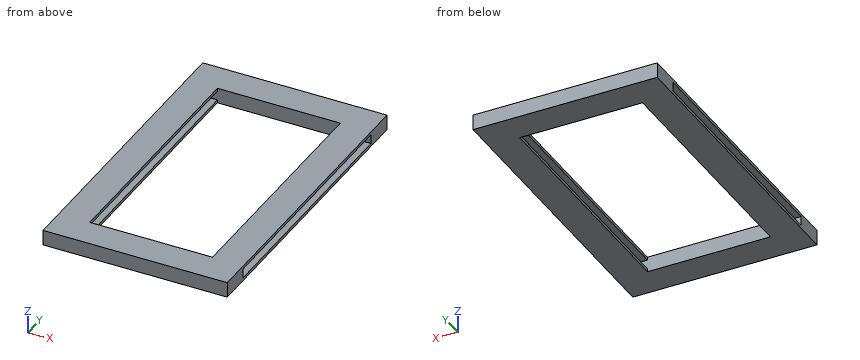
from build123d import *

# Parameters (mm, degrees)
CROQUIS1_W              = 60
CROQUIS1_H              = 100
SALIENTE_EXTRUIR1_DEPTH = 5
CROQUIS3_W              = 3
CROQUIS3_H              = 80
CORTAR_EXTRUIR2_DEPTH   = 60
CROQUIS4_W              = 40
CROQUIS4_H              = 80
CORTAR_EXTRUIR3_DEPTH   = 28


with BuildPart() as part:
    # Croquis1 → Saliente-Extruir1 (new body)
    with BuildSketch(Plane.XY):
        with Locations((-30, 50)):
            Rectangle(CROQUIS1_W, CROQUIS1_H)
    extrude(amount=SALIENTE_EXTRUIR1_DEPTH)

    # Croquis3 → Cortar-Extruir2 (cut)
    with BuildSketch(Plane.ZY.offset(60)):
        with Locations((2.5, 50)):
            Rectangle(CROQUIS3_W, CROQUIS3_H)
    extrude(amount=-CORTAR_EXTRUIR2_DEPTH, mode=Mode.SUBTRACT)

    # Croquis4 → Cortar-Extruir3 (cut)
    with BuildSketch(Plane(origin=(0, 0, 0), x_dir=(-1, 0, 0), z_dir=(0, 0, -1))):
        with Locations((30, 50)):
            Rectangle(CROQUIS4_W, CROQUIS4_H)
    extrude(amount=-CORTAR_EXTRUIR3_DEPTH, mode=Mode.SUBTRACT)


solid = part.part
Geometry: final body of the model. Coordinates: model frame, mm. Give positions to 0.01 mm unless a question says otherwise; leave off trailing zeros. Write each loop counter-clockwise with the first axis right and the second up, starting at its lowest first coordinate (ties: lowest second). Pieces come first, ordered by that corner, then holes.
(1) Cut plane A-A, the plane z = 2.6. Return loops of the section in (x, y).
(2) Cut plane B-B, the plane x = -49. Return loops of the section in (y, z), then the cut area to 3 significant figures.
(3) Cut plane C-C, the plane y = 75. Return loops of the section in (x, z), then the cut area to 3 significant figures.
(4) Ray query, line 1 (Y direction, x = -34, z = 1.5); line 2 (Z direction, x = -5.5, y = 14.5); line 3 (X direction, y = 48, z = 0.35). Return the intervals inside material, ascending.
Values follow:
1. outline: (-60, 0) - (0, 0) - (0, 10) - (-60, 10) - close; (-60, 90) - (0, 90) - (0, 100) - (-60, 100) - close
2. outline: (0, 0) - (10, 0) - (10, 5) - (0, 5) - close; (90, 0) - (100, 0) - (100, 5) - (90, 5) - close
2. area: 100 mm2
3. outline: (-60, 0) - (-50, 0) - (-50, 1) - (-60, 1) - close; (-60, 4) - (-50, 4) - (-50, 5) - (-60, 5) - close; (-10, 0) - (0, 0) - (0, 1) - (-10, 1) - close; (-10, 4) - (0, 4) - (0, 5) - (-10, 5) - close
3. area: 40.0 mm2
4. line 1: y = 0 to 10, 90 to 100
4. line 2: z = 0 to 1, 4 to 5
4. line 3: x = -60 to -50, -10 to 0
